from build123d import *

# Parameters (mm, degrees)
SKETCH2_W           = 55
SKETCH2_H           = 13.45
BOSS_EXTRUDE1_DEPTH = 12.2
SKETCH3_W           = 18.5
SKETCH3_H           = 10.25
CUT_EXTRUDE1_DEPTH  = 7.6
SKETCH5_W           = 22.15
SKETCH5_H           = 1.6
CUT_EXTRUDE2_DEPTH  = 4
SKETCH6_W           = 17.75
SKETCH6_H           = 2
BOSS_EXTRUDE2_DEPTH = 8.7
SKETCH7_W           = 1.825
SKETCH7_H           = 3.375
CUT_EXTRUDE3_DEPTH  = 4
FILLET1_R           = 0.75
FILLET3_R           = 0.75
DRAFT4_ANGLE        = 60
FILLET5_R           = 6
SKETCH8_R           = 2.5
CUT_EXTRUDE4_DEPTH  = 58.328314378
SKETCH9_R           = 4.25
CUT_EXTRUDE5_DEPTH  = 3
SKETCH10_R          = 5.3
CUT_EXTRUDE6_DEPTH  = 3.15
CUT_EXTRUDE7_DEPTH  = 11
FILLET6_R           = 1.5


with BuildPart() as part:
    # Sketch2 → Boss-Extrude1 (new body)
    with BuildSketch(Plane.XY):
        with Locations((27.5, 6.725)):
            Rectangle(SKETCH2_W, SKETCH2_H)
    extrude(amount=BOSS_EXTRUDE1_DEPTH)

    # Sketch3 → Cut-Extrude1 (cut)
    with BuildSketch(Plane.XY.offset(12.2)):
        with Locations((27.5, 6.725)):
            Rectangle(SKETCH3_W, SKETCH3_H)
    extrude(amount=-CUT_EXTRUDE1_DEPTH, mode=Mode.SUBTRACT)

    # Sketch5 → Cut-Extrude2 (cut)
    with BuildSketch(Plane.XY.offset(12.2)):
        with Locations((27.5, 12.65)):
            Rectangle(SKETCH5_W, SKETCH5_H)
    extrude(amount=-CUT_EXTRUDE2_DEPTH, mode=Mode.SUBTRACT)

    # Sketch6 → Boss-Extrude2 (add)
    with BuildSketch(Plane.XY.offset(12.2)):
        with Locations((27.5, 13.275)):
            Rectangle(SKETCH6_W, SKETCH6_H)
    extrude(amount=-BOSS_EXTRUDE2_DEPTH)

    # Sketch7 → Cut-Extrude3 (cut)
    with BuildSketch(Plane.XY.offset(12.2)):
        with Locations((37.6625, 11.7625)):
            Rectangle(SKETCH7_W, SKETCH7_H)
        with Locations((17.3375, 11.7625)):
            Rectangle(SKETCH7_W, SKETCH7_H)
    extrude(amount=-CUT_EXTRUDE3_DEPTH, mode=Mode.SUBTRACT)

    # Fillet1
    fillet1_edges = [part.edges().sort_by_distance(p)[0] for p in [
        (36.375, 14.275, 7.85),
        (36.375, 12.275, 10.2),
    ]]
    fillet(fillet1_edges, radius=FILLET1_R)

    # Fillet3
    fillet3_edges = [part.edges().sort_by_distance(p)[0] for p in [
        (18.625, 12.275, 10.2),
        (18.625, 14.275, 7.85),
    ]]
    fillet(fillet3_edges, radius=FILLET3_R)

    # Draft4
    draft4_faces = [part.faces().sort_by_distance(p)[0] for p in [
        (27.5, 13.858393484, 3.5),
    ]]
    draft(draft4_faces, Plane(origin=(18.625, 14.275, 3.5), x_dir=(0, 0, 1), z_dir=(0, 1, 0)), DRAFT4_ANGLE)

    # Fillet5
    # the kernel refuses this fillet: 6 mm, written as the material it takes off along each edge
    with BuildSketch(Plane(origin=(39.644237886, 14.275, 3.5), x_dir=(0, -0.49999999999999806, -0.8660254037844397), z_dir=(-1, 0, 0))) as fillet5_piece_1:
        with BuildLine():
            CenterArc((FILLET5_R * 0.267949192431, FILLET5_R), FILLET5_R, 240, 30)
            Line((-FILLET5_R * 0.232050807569, FILLET5_R * 0.133974596216), (0, 0))
            Line((0, 0), (FILLET5_R * 0.267949192431, 0))
        make_face()
    extrude(amount=24.288475773, mode=Mode.SUBTRACT)

    # Sketch8 → Cut-Extrude4 (cut, through all)
    with BuildSketch(Plane.XY.offset(4.6)):
        with Locations((27.5, 6.725)):
            Circle(SKETCH8_R)
    extrude(amount=-CUT_EXTRUDE4_DEPTH, mode=Mode.SUBTRACT)

    # Sketch9 → Cut-Extrude5 (cut)
    with BuildSketch(Plane(origin=(0, 0, 0), x_dir=(-1, 0, 0), z_dir=(0, 0, -1))):
        with Locations((-27.5, 6.725)):
            Circle(SKETCH9_R)
    extrude(amount=-CUT_EXTRUDE5_DEPTH, mode=Mode.SUBTRACT)

    # Sketch10 → Cut-Extrude6 (cut)
    with BuildSketch(Plane(origin=(0, 0, 0), x_dir=(-1, 0, 0), z_dir=(0, 0, -1))):
        with Locations((-48, 6.725)):
            Circle(SKETCH10_R)
        with Locations((-7, 6.725)):
            Circle(SKETCH10_R)
    extrude(amount=-CUT_EXTRUDE6_DEPTH, mode=Mode.SUBTRACT)

    # Sketch11 → Cut-Extrude7 (cut)
    with BuildSketch(Plane(origin=(0, 13.45, 0), x_dir=(1, 0, 0), z_dir=(0, 1, 0))):
        Polygon((9.020725942, -3.15), (4.979274058, -3.15), (2.958548116, -6.65), (4.979274058, -10.15), (9.020725942, -10.15), (11.041451884, -6.65), align=None)
        Polygon((43.958548116, -6.65), (45.979274058, -3.15), (50.020725942, -3.15), (52.041451884, -6.65), (50.020725942, -10.15), (45.979274058, -10.15), align=None)
    extrude(amount=-CUT_EXTRUDE7_DEPTH, mode=Mode.SUBTRACT)

    # Fillet6
    fillet6_edges = [part.edges().sort_by_distance(p)[0] for p in [
        (55, 6.725, 12.2),
        (0, 6.725, 12.2),
        (55, 6.725, 0),
        (0, 6.725, 0),
    ]]
    fillet(fillet6_edges, radius=FILLET6_R)


solid = part.part
Read the model definition and answer for the solid it produces. Units are mm, in the model's axes. A direction names the side the tool comes from. Coordinates: 2 decimals unless noted, no trailing zeros. Loops run counter-clockwise (first coordinate to the right, second up) from the corner with the lowest first, then second, coordinate; pieces in that order, holes last.
Q1. Each of these flat-tipped pins is pushed along its axis until it touches: pin 1 Ø2 at (x, y) = (14, 4.5) entering from -Z; pin 2 Ø0.5 at (x, z) = (37.5, 10) entering from +Y (3 decimals); pin 3 Ø5 at (x, y) = (7.5, 7) entering from -Z; pin 4 Ø2 at (x, z) = (47.5, 6) entering from +Y. Where does it stop, or does it pass through?
Q2. The part is cut by section C-C on z = 11.5. Write down the section's boundary in (x, y) (3 decimals), and give its area (3 significant figures).
Q3. The part is cut by section D-D on x = 27.5. Write down the section's boundary in (y, z) (3 decimals).
Q4. The part is cut by section B-B on z = 7.5. Write down the section's boundary in (x, y) (3 decimals).
Q5. The part is cut by section A-A on x = 48. Write down the section's boundary in (y, z) (3 decimals), and give its area (3 significant figures).
Q6. Consider probe 1 along Y at (x, z) = (7, 0.9) (3 decimals); probe 2 along Y at (x, z) = (27.5, 0.8) (3 decimals); probe 3 along X at (y, z) = (11, 4.25). Determine where each line is inside the solid, lowest interval first.
Q7. Which of the six approach directions +Z, -Z, +X, -X, +Y, -Y give full straight-line access (tool end or side, diameter ignored) to faces 4 (the face through (17, 10.075, 10)), 5 (the face through (27, 1.6, 8)), 6 (the face through (4.7, 6.6, 3.15)), 7 (the face through (44.955, 8.027, 4.924))?
Q8. The mould has two halves that part along Y. Classify faces 1 (the face through (48, 2.45, 7)), 2 (the face through (7, 8, 10.15)), 3 (the face through (45.7, 6.6, 3.15)): +Y half, -Y half, draft (parallel to the pull), parting line (faces both ways), or undercut.
Results below:
1. pin 1: stops at z = 0
1. pin 2: stops at y = 10.075
1. pin 3: stops at z = 3.15
1. pin 4: stops at y = 2.45
2. outline: (0.231, 0) - (54.769, 0) - (54.769, 13.45) - (38.575, 13.45) - (38.575, 10.075) - (36.75, 10.075) - (36.75, 1.6) - (18.25, 1.6) - (18.25, 10.075) - (16.425, 10.075) - (16.425, 13.45) - (0.231, 13.45) - close; (18.625, 13.025) arc R0.75 ccw to (19.375, 12.275) - (35.625, 12.275) arc R0.75 ccw to (36.375, 13.025) - (36.375, 13.525) arc R0.75 ccw to (35.625, 14.275) - (19.375, 14.275) arc R0.75 ccw to (18.625, 13.525) - close
2. area: 537 mm2
3. outline: (0, 0) - (2.475, 0) - (2.475, 3) - (4.225, 3) - (4.225, 4.6) - (1.6, 4.6) - (1.6, 12.2) - (0, 12.2) - close; (9.225, 3) - (10.975, 3) - (10.975, 0) - (13.45, 0) - (13.45, 2.071) - (13.471, 2.108) arc R6 ccw to (14.275, 5.108) - (14.275, 12.2) - (12.275, 12.2) - (12.275, 8.2) - (11.85, 8.2) - (11.85, 4.6) - (9.225, 4.6) - close
4. outline: (0, 0) - (55, 0) - (55, 13.45) - (51.551, 13.45) - (51.551, 2.45) - (44.449, 2.45) - (44.449, 13.45) - (36.375, 13.45) - (36.375, 13.525) arc R0.75 ccw to (35.625, 14.275) - (19.375, 14.275) arc R0.75 ccw to (18.625, 13.525) - (18.625, 13.45) - (10.551, 13.45) - (10.551, 2.45) - (3.449, 2.45) - (3.449, 13.45) - (0, 13.45) - close; hole (18.25, 1.6) - (36.75, 1.6) - (36.75, 11.85) - (18.25, 11.85) - close
5. outline: (0, 0) - (1.425, 0) - (1.425, 3.15) - (2.45, 3.15) - (2.45, 10.15) - (13.45, 10.15) - (13.45, 12.2) - (0, 12.2) - close; (12.025, 0) - (13.45, 0) - (13.45, 3.15) - (12.025, 3.15) - close
5. area: 53.7 mm2
6. probe 1: y = 0 to 1.425, 12.025 to 13.45
6. probe 2: y = 0 to 2.475, 10.975 to 13.45
6. probe 3: x = 0 to 4.34, 9.66 to 45.34, 50.66 to 55
7. face 4: +Z, +Y
7. face 5: +Z
7. face 6: -Z
7. face 7: +Y
8. face 1: +Y half
8. face 2: draft
8. face 3: undercut
